Design review of the part built by this model. Coordinates are the model's own, in mm. A direction names the side the tool comes from. Coordinates: 2 decimals unless noted, no trailing zeros. Loops run counter-clockwise (first coordinate to the right, second up) from the corner with the lowest first, then second, coordinate; pieces in that order, holes last.
Q1. Add section B-B on x = 35.5. Give the boundary of the cut face in (y, z), and give its area (3 significant figures).
Q2. Add section A-A on y = 231. Give the boundary of the cut face in (x, z).
Q3. Machinability: for faces 1 (the face through (0, 554, 207)), 2 (the face through (275, 0, 207)), 3 (the face through (609, 247.65, 207)), 4 (the face through (335, 1092.2, 207)), 5 (the face through (628.65, 537, -72)), which of the approach directions +Z, -Z, +X, -X, +Y, -Y give a long, thin tool a straight path to every point of the face, cutting with its end or side? Answer none if there is none.
Q4. Add section D-D on z = -46.5. Give the boundary of the cut face in (x, y).
Q5. Wall thickness on probe 1 along Z at (x, y) = (-24, 169.5); probe 2 along X at (y, z) = (864, -88.5); probe 3 along Y at (x, z) = (240, 40): over which ranges is each line inside the solid? List them lowest first.
Q6. Add section C-C on z = 357. Give the boundary of the cut face in (x, y), and give its area (3 significant figures).
Q7. For P1, Ø2, axis at x = 335, z = 38, coming from the +Y side; P2, Ø8, axis at y = 174, z = 235.5, coming from the +X side; P3, Ø1, axis at y = 102, z = 295.5, coming from the -X side, all flat-tipped, find the tip position at first contact; note any pin that passes through.
```python
from build123d import *

# Parameters (mm, degrees)
F1_DEPTH = 419.1
F3_DEPTH = 146.05


with BuildPart() as f1:
    # F0 (on Top) → F1 (new body)
    with BuildSketch(Plane.XY):
        Polygon((0, 1092.2), (0, 0), (558.8, 0), (558.8, 247.65), (660.4, 247.65), (660.4, 1092.2), (558.8, 1092.2), align=None)
    extrude(amount=F1_DEPTH)

    # F2 (on Top) → F3 (join)
    with BuildSketch(Plane.XY):
        Polygon((628.65, 1162.05), (-69.85, 1162.05), (-69.85, -69.85), (628.65, -69.85), (628.65, 133.35), (628.65, 958.85), align=None)
    extrude(amount=-F3_DEPTH)


solid = f1.part
```
Entries:
1. outline: (-69.85, -146.05) - (1162.05, -146.05) - (1162.05, 0) - (1092.2, 0) - (1092.2, 419.1) - (0, 419.1) - (0, 0) - (-69.85, 0) - close
1. area: 638,000 mm2
2. outline: (-69.85, -146.05) - (628.65, -146.05) - (628.65, 0) - (558.8, 0) - (558.8, 419.1) - (0, 419.1) - (0, 0) - (-69.85, 0) - close
3. face 1: +Z, -X, +Y, -Y
3. face 2: +Z, +X, -X, -Y
3. face 3: +Z, +X, -Y
3. face 4: +Z, +X, -X, +Y
3. face 5: -Z, +X, +Y, -Y
4. outline: (-69.85, -69.85) - (628.65, -69.85) - (628.65, 1162.05) - (-69.85, 1162.05) - close
5. probe 1: z = -146.05 to 0
5. probe 2: x = -69.85 to 628.65
5. probe 3: y = 0 to 1092.2
6. outline: (0, 0) - (558.8, 0) - (558.8, 247.65) - (660.4, 247.65) - (660.4, 1092.2) - (0, 1092.2) - close
6. area: 696,000 mm2
7. P1: stops at y = 1092.2
7. P2: stops at x = 558.8
7. P3: stops at x = 0
